Check sheet for the drawn part. Datum: minimum x, y, z corner. Units: mm. Give positions to 0.01 mm unless a question says otherwise; leave off trailing zeros.
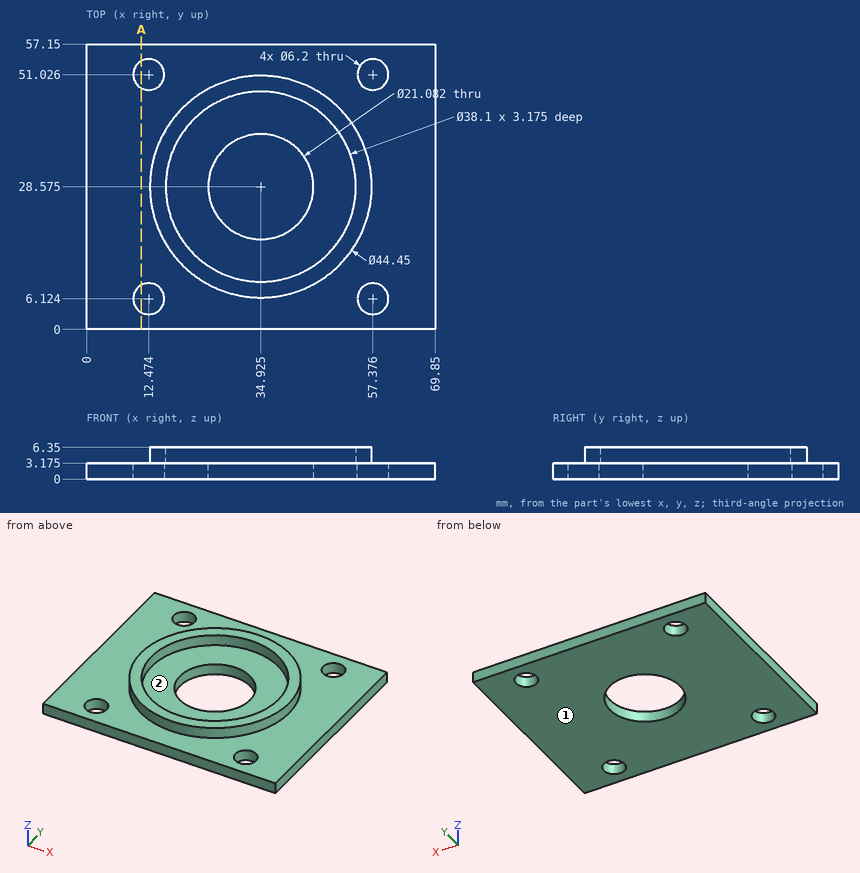
(1) Scan lines: line 1 (Y direction, x = 57, z = 1.5); line 2 (X direction, y = 51.5, z = 3); line 3 (X direction, y = 42, z = 5.5) (1 decimal). Record each from-to range of solid material in increasing order.
Solved:
line 1: y = 0 to 3.05, 9.2 to 47.95, 54.1 to 57.15
line 2: x = 0 to 9.41, 15.54 to 54.31, 60.44 to 69.85
line 3: x = 17.2 to 21.4, 48.4 to 52.6
(2) Release check for a two-part mould opening along Y. For the marked faces 1 and 2 record: pulls with the +Y half, pulls with the -Y half, needs draft (parallel to the pull), parting line crosses it, or undercut.
Solved:
face 1: needs draft
face 2: undercut
(3) Section check A-A, the plane x = 11. Give the number of separate pieces and of enclosed holes in the cut face, then the cut area to 3 significant figures.
Solved:
separate pieces: 3
enclosed holes: 0
area: 147 mm2
(4) Go/stop test with flat-tipped pins: pin 1 (7 mm diameter, centred on x = 57.38, y = 51.03, fed in from +Z) (3 decimals); pin 2 (5 mm diameter, centred on x = 12.47, y = 6.12, fed in from +Z). Record where each tip stops, or that it passes through.
Solved:
pin 1: stops at z = 3.175
pin 2: passes through
